Verification items for the finished model (mm, model axes). Face numbers are marked on the shaded views. A direction names the side the tool comes from. Coordinates: 2 decimals unless noted, no trailing zeros. Order: outer loops, then holes, each group sorted by start corner. A loop starts at its lowest first (then second) coordinate and runs counter-clockwise, first axis right, second up. Notation, with made-up numbers: (39, 86.5) -> (61, 86.5) arc R11 cw to (61, 94.5) -> close; hole circle Ø6 at (45, 84). An arc over 180 degrees is marked (long way). Write each question's results on one line, items separated by ' | '. Start each with the question number.
(1) Thickness scan on probe 1 along Y at (x, z) = (-218, 2.75); probe 2 along Y at (x, z) = (-191, -3); probe 3 along X at (y, z) = (-471.5, -14.5). Record the ranges inside material, lowest first. Write a range as [from, to].
(2) Draft check along Y on the marked faces 3, 4 and 5. Enter one of: +Y half, -Y half, draft (parallel to the pull), parting line (faces both ways), or undercut.
(3) Cross-section at C-C on z = -0.75. Enter the section's corners in (x, y), and give its area (3 significant figures).
(4) Cross-section at A-A on z = -10. Enter the section's corners in (x, y), and give its area (3 significant figures).
(5) Go/stop test with flat-tipped pins: pin 1 (5 mm diameter, centred on x = -195, z = -5, fed in from -Y); pin 2 (6.5 mm diameter, centred on y = -511.28, z = -10, fed in from +X); pin 3 (12 mm diameter, centred on x = -199, z = -3, fed in from -Y); pin 4 (5 mm diameter, centred on x = -218.5, y = -507, fed in from -Z). Record where each tip stops, or that it passes through.
(6) Set-up check for the marked faces 1 and 2: record each of +Z, -Z, +X, -X, +Y, -Y from which the full face is reachable in a straight line by a thin tool's end or side.
(7) Cross-section at B-B on x = -218.5. Enter the section's corners in (y, z).
(8) Cross-section at D-D on y = -495.5. Enter the section's corners in (x, z).
```python
from build123d import *

# Parameters (mm, degrees)
SKETCH1_W           = 40
SKETCH1_H           = 70
SKETCH1_R           = 2.74
BOSS_EXTRUDE1_DEPTH = 4
SKETCH2_W           = 40
SKETCH2_H           = 24
SKETCH2_R           = 2.74
BOSS_EXTRUDE2_DEPTH = 4
SKETCH3_W           = 24
SKETCH3_H           = 74
SKETCH3_R           = 2.74
BOSS_EXTRUDE3_DEPTH = 4


with BuildPart() as part:
    # Sketch1 → Boss-Extrude1 (new body)
    with BuildSketch(Plane.XY):
        with Locations((-209.068179547, -486.277483232)):
            Rectangle(SKETCH1_W, SKETCH1_H)
        with Locations((-199.068179547, -461.277483232)):
            Circle(SKETCH1_R, mode=Mode.SUBTRACT)
        with Locations((-219.139101533, -461.277483232)):
            Circle(SKETCH1_R, mode=Mode.SUBTRACT)
        with Locations((-219.139101533, -511.277483232)):
            Circle(SKETCH1_R, mode=Mode.SUBTRACT)
        with Locations((-199.068179547, -511.277483232)):
            Circle(SKETCH1_R, mode=Mode.SUBTRACT)
    extrude(amount=BOSS_EXTRUDE1_DEPTH)

    # Sketch2 → Boss-Extrude2 (add)
    with BuildSketch(Plane(origin=(0, -451.277483232, 0), x_dir=(1, 0, 0), z_dir=(0, 1, 0))):
        with Locations((-209.068179547, 8)):
            Rectangle(SKETCH2_W, SKETCH2_H)
        with Locations(Location((-199.068179547, 10, 0), (0, 0, 270))):
            Circle(SKETCH2_R, mode=Mode.SUBTRACT)
    extrude(amount=BOSS_EXTRUDE2_DEPTH)

    # Sketch3 → Boss-Extrude3 (add)
    with BuildSketch(Plane.ZY.offset(229.068179547)):
        with Locations((-8, -484.277483232)):
            Rectangle(SKETCH3_W, SKETCH3_H)
        with Locations(Location((-10, -461.277483232, 0), (0, 0, 270))):
            Circle(SKETCH3_R, mode=Mode.SUBTRACT)
        with Locations(Location((-10, -511.277483232, 0), (0, 0, 270))):
            Circle(SKETCH3_R, mode=Mode.SUBTRACT)
    extrude(amount=BOSS_EXTRUDE3_DEPTH)


solid = part.part
```
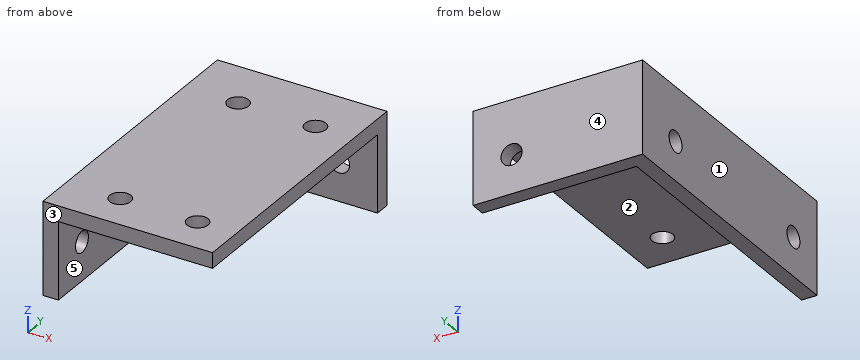
Results are:
1) probe 1: y = [-521.28, -513.77], [-508.79, -463.77], [-458.79, -447.28] | probe 2: y = [-451.28, -447.28] | probe 3: x = [-233.07, -229.07]
2) face 3: -Y half | face 4: +Y half | face 5: draft
3) outline: (-233.07, -521.28) -> (-229.07, -521.28) -> (-229.07, -451.28) -> (-189.07, -451.28) -> (-189.07, -447.28) -> (-233.07, -447.28) -> close | area: 456 mm2
4) outline: (-233.07, -521.28) -> (-229.07, -521.28) -> (-229.07, -514.02) -> (-233.07, -514.02) -> close; (-233.07, -508.54) -> (-229.07, -508.54) -> (-229.07, -464.02) -> (-233.07, -464.02) -> close; (-233.07, -458.54) -> (-229.07, -458.54) -> (-229.07, -451.28) -> (-201.81, -451.28) -> (-201.81, -447.28) -> (-233.07, -447.28) -> close; (-196.33, -451.28) -> (-189.07, -451.28) -> (-189.07, -447.28) -> (-196.33, -447.28) -> close | area: 390 mm2
5) pin 1: stops at y = -451.28 | pin 2: stops at x = -229.07 | pin 3: stops at y = -521.28 | pin 4: stops at z = 0
6) face 1: +Z, -Z, -X, +Y, -Y | face 2: -Z, +X, -Y
7) outline: (-521.28, 0) -> (-513.94, 0) -> (-513.94, 4) -> (-521.28, 4) -> close; (-508.61, 0) -> (-463.94, 0) -> (-463.94, 4) -> (-508.61, 4) -> close; (-458.61, 0) -> (-451.28, 0) -> (-451.28, -20) -> (-447.28, -20) -> (-447.28, 4) -> (-458.61, 4) -> close
8) outline: (-233.07, -20) -> (-229.07, -20) -> (-229.07, 0) -> (-189.07, 0) -> (-189.07, 4) -> (-233.07, 4) -> close
